Can you work these out from the drawing? Everything is in mm from the part's minimum corner. Coordinates: 2 decimals unless noted, no trailing zeros. Loops run counter-clockwise (first coordinate to the right, second up) from the corner with the lowest first, then second, coordinate; pieces in that order, holes last.
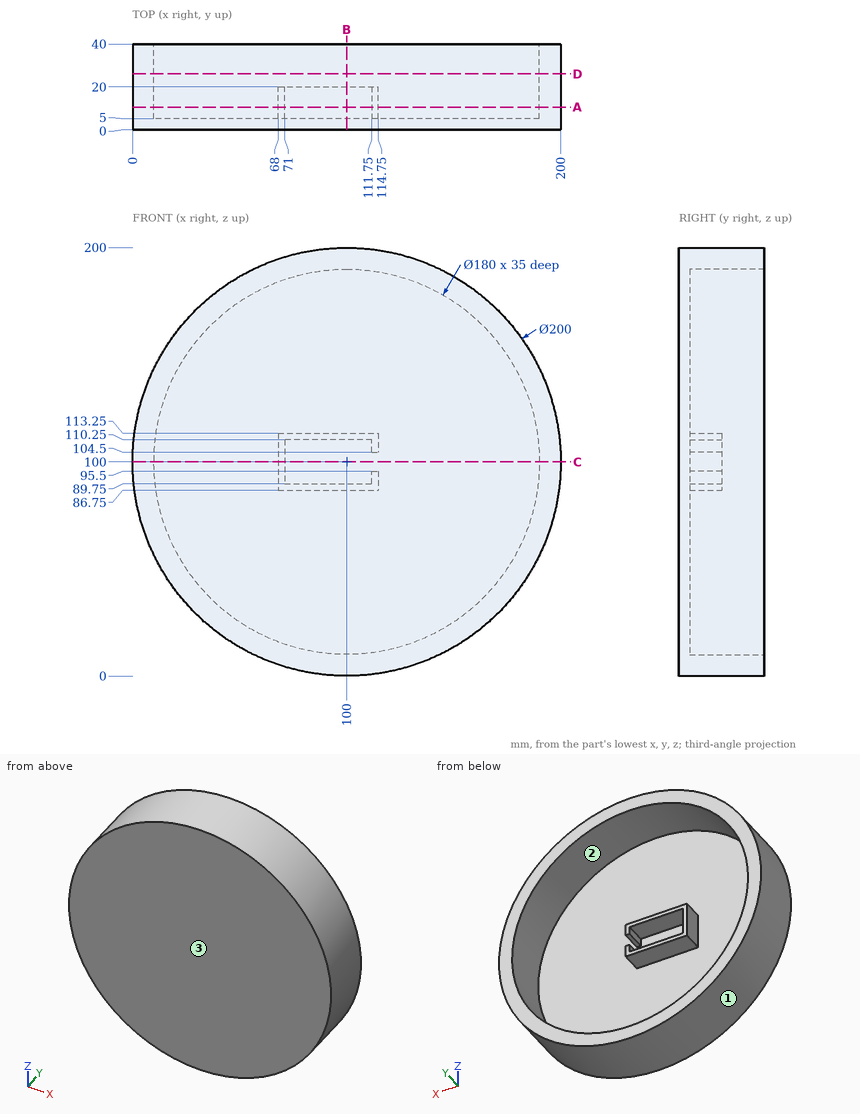
(1) We'd pull the mould along Z, two halves only. Please class the marked faces 1, 2 and 3: +Z half, -Z half, draft (parallel to the pull), parting line (faces both ways), or undercut.
Answers:
face 1: parting line
face 2: undercut
face 3: draft
(2) Imagine slicing it at C-C, the plane z = 100. Write out the boundary of the cut face in (x, y).
Answers:
outline: (0, 0) - (200, 0) - (200, 40) - (190, 40) - (190, 5) - (71, 5) - (71, 20) - (68, 20) - (68, 5) - (10, 5) - (10, 40) - (0, 40) - close
(3) I need wall thicknesses on probe 1 along X at (y, z) = (23, 100); probe 2 along Z at (x, y) = (103.5, 11); probe 3 along Y at (x, z) = (132, 168). Which ranges of each line are inside material? Lowest first, please.
Answers:
probe 1: x = 0 to 10, 190 to 200
probe 2: z = 0.06 to 10.07, 86.75 to 89.75, 110.25 to 113.25, 189.93 to 199.94
probe 3: y = 0 to 5
(4) Imagine slicing it at B-B, the plane x = 100. Write out the boundary of the cut face in (y, z), and give its area (3 significant figures).
Answers:
outline: (0, 0) - (40, 0) - (40, 10) - (5, 10) - (5, 86.75) - (20, 86.75) - (20, 89.75) - (5, 89.75) - (5, 110.25) - (20, 110.25) - (20, 113.25) - (5, 113.25) - (5, 190) - (40, 190) - (40, 200) - (0, 200) - close
area: 1,790 mm2
(5) For pin 1 (9.5 mm diameter, centred on y = 16, z = 91.5, fed in from +X); pin 2 (3.5 mm diameter, centred on x = 112.5, y = 14, fed in from -Z); pin 3 (2 mm diameter, centred on x = 128, y = 5.5, fed in from +Z), each with a flat end and sliding along its axis, tell me the tip position at first contact or that it passes through.
Answers:
pin 1: stops at x = 199.93
pin 2: stops at z = 0.58
pin 3: stops at z = 196.29
(6) Imagine slicing it at A-A, the plane y = 10.5. Write out the boundary of the cut face in (x, z).
Answers:
outline: circle Ø200 at (100, 100); (68, 86.75) - (114.75, 86.75) - (114.75, 95.5) - (111.75, 95.5) - (111.75, 89.75) - (71, 89.75) - (71, 110.25) - (111.75, 110.25) - (111.75, 104.5) - (114.75, 104.5) - (114.75, 113.25) - (68, 113.25) - close; hole circle Ø180 at (100, 100)
(7) Imagine slicing it at D-D, the plane y = 26. Write out the boundary of the cut face in (x, z).
Answers:
outline: circle Ø200 at (100, 100); hole circle Ø180 at (100, 100)
